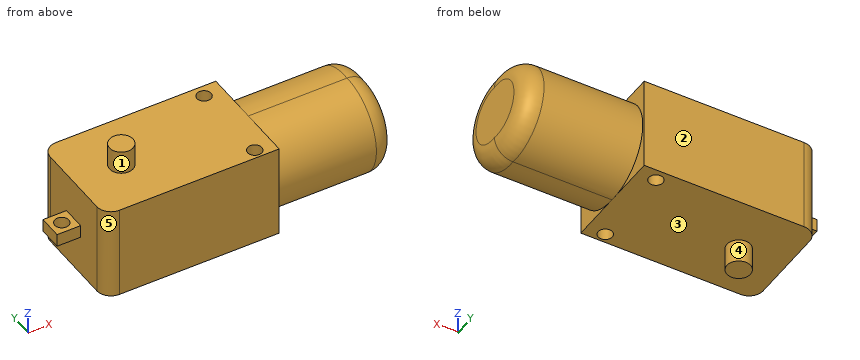
from build123d import *

# Parameters (mm, degrees)
SKETCH1_W           = 37
SKETCH1_H           = 22.5
BOSS_EXTRUDE1_DEPTH = 20
BOSS_EXTRUDE2_DEPTH = 25
SKETCH3_R           = 2.5
BOSS_EXTRUDE3_DEPTH = 5
BOSS_EXTRUDE4_START = 5
SKETCH4_R           = 2.5
BOSS_EXTRUDE4_DEPTH = 5
FILLET1_R           = 3
FILLET2_R           = 4
SKETCH5_W           = 2.75
SKETCH5_H           = 5
BOSS_EXTRUDE5_DEPTH = 5
SKETCH6_R           = 1.5
CUT_EXTRUDE1_DEPTH  = 2.75
SKETCH7_R           = 1.5
CUT_EXTRUDE2_DEPTH  = 78.76577433


with BuildPart() as part:
    # Sketch1 → Boss-Extrude1 (new body)
    with BuildSketch(Plane.XY):
        with Locations((-45.764100782, -13.75)):
            Rectangle(SKETCH1_W, SKETCH1_H)
    extrude(amount=-BOSS_EXTRUDE1_DEPTH)

    # Sketch2 → Boss-Extrude2 (add)
    with BuildSketch(Plane(origin=(-27.264100782, 0, 0), x_dir=(0, 0, -1), z_dir=(1, 0, 0))):
        with BuildLine():
            ThreePointArc((0.050125629, -14), (10, -24.462429423), (19.949874371, -14))
            ThreePointArc((19.949874371, -14), (10, -3), (0.050125629, -14))
        make_face()
    extrude(amount=BOSS_EXTRUDE2_DEPTH)

    # Sketch3 → Boss-Extrude3 (add)
    with BuildSketch(Plane.XY):
        with Locations((-54.264100782, -14)):
            Circle(SKETCH3_R)
    extrude(amount=BOSS_EXTRUDE3_DEPTH)

    # Sketch4 → Boss-Extrude4 (add)
    with BuildSketch(Plane(origin=(0, 0, -20), x_dir=(-1, 0, 0), z_dir=(0, 0, -1)).offset(BOSS_EXTRUDE4_START)):
        with Locations(Location((54.264100782, -14, 0), (0, 0, 180))):
            Circle(SKETCH4_R)
    extrude(amount=-BOSS_EXTRUDE4_DEPTH)

    # Fillet1
    fillet1_edges = [part.edges().sort_by_distance(p)[0] for p in [
        (-64.264100782, -2.5, -10),
        (-64.264100782, -25, -10),
    ]]
    fillet(fillet1_edges, radius=FILLET1_R)

    # Fillet2
    fillet2_edges = [part.edges().sort_by_distance(p)[0] for p in [
        (-2.264100782, -3, -10),
        (-2.264100782, -24.462429423, -10),
    ]]
    fillet(fillet2_edges, radius=FILLET2_R)

    # Sketch5 → Boss-Extrude5 (add)
    with BuildSketch(Plane.ZY.offset(64.264100782)):
        with Locations((-10, -13.75)):
            Rectangle(SKETCH5_W, SKETCH5_H)
    extrude(amount=BOSS_EXTRUDE5_DEPTH)

    # Sketch6 → Cut-Extrude1 (cut)
    with BuildSketch(Plane(origin=(0, 0, -11.375), x_dir=(-1, 0, 0), z_dir=(0, 0, -1))):
        with Locations((66.764100782, -13.75)):
            Circle(SKETCH6_R)
    extrude(amount=-CUT_EXTRUDE1_DEPTH, mode=Mode.SUBTRACT)

    # Sketch7 → Cut-Extrude2 (cut, through all)
    with BuildSketch(Plane(origin=(0, 0, -20), x_dir=(-1, 0, 0), z_dir=(0, 0, -1))):
        with Locations((31.264100782, -5)):
            Circle(SKETCH7_R)
        with Locations((31.264100782, -23)):
            Circle(SKETCH7_R)
    extrude(amount=-CUT_EXTRUDE2_DEPTH, mode=Mode.SUBTRACT)


solid = part.part
Verification items for the finished model (mm, model axes). Face numbers are marked on the shaded views. A direction names the side the tool comes from. Give positions to 0.01 mm unless a question says otherwise; leave off trailing zeros. Order: outer loops, then holes, each group sorted by start corner. A loop starts at its lowest first (then second) coordinate and runs counter-clockwise, first axis right, second up. Notation, with made-up numbers: M 71.25,13.25 L 77.25,13.25 A18 cw 77.25,34.25 Z; hole C 51,-24.75 d5. An arc over 180 degrees is marked long. Use one line per item in the form item = value. Start each with the question number.
Q1. Section check A-A (z = -10). Enter the section's corners in (x, y).
Q2. Mould release check, pull along X, two halves, no side actions. Record for the marked faces 3, 4 and 5: +X half, -X half, draft (parallel to the pull), parting line (faces both ways), or undercut.
Q3. Scan lines: line 1 along Z through (x, y) = (-38.5, -12); line 2 along X through (y, z) = (-13.25, -3.75); line 3 along Z through (x, y) = (-16.5, -14). Record each from-to range of solid material in increasing order. Write a range as [from, to].
Q4. Section check C-C (z = -15). Count the separate pieces of the cut face and the enclosed holes in it, then the cut area to 3 significant figures.
Q5. Access from +Z, -Z, +X, -X, +Y, -Y to the whole of each face (thin tool, end or side, straight path). Record for the marked faces 1 and 2.
Q6. Section check B-B (x = -60). Enter the section's corners in (y, z), then the cut area to 3 significant figures.
Q7. Section check D-D (z = 2.75). Enter the section's corners in (x, y).
Q8. Go/stop test with flat-tipped pins: pin 1 Ø3.5 at (x, y) = (-66.76, -13.75) entering from -Z (3 decimals); pin 2 Ø1 at (y, z) = (-6, -15) entering from -X; pin 3 Ø3 at (x, z) = (-67.5, -10) entering from -Y. Record where each tip stops, or that it passes through.
Evaluation:
q1.outline = M -69.26,-16.25 L -64.26,-16.25 L -64.26,-22 A3 ccw -61.26,-25 L -27.26,-25 L -27.26,-24.46 L -6.26,-24.46 A4 ccw -2.26,-20.46 L -2.26,-7 A4 ccw -6.26,-3 L -27.26,-3 L -27.26,-2.5 L -61.26,-2.5 A3 ccw -64.26,-5.5 L -64.26,-11.25 L -69.26,-11.25 Z; hole C -66.76,-13.75 d3; hole C -31.26,-23 d3; hole C -31.26,-5 d3
q2.face_3 = draft
q2.face_4 = parting line
q2.face_5 = -X half
q3.line_1 = [-20, 0]
q3.line_2 = [-64.26, -2.27]
q3.line_3 = [-19.95, -0.05]
q4.separate_pieces = 1
q4.enclosed_holes = 2
q4.area = 1,280 mm2
q5.face_1 = +Z
q5.face_2 = +Z, -Z, +X, -X, +Y
q6.outline = M -25,-20 L -2.5,-20 L -2.5,0 L -25,0 Z
q6.area = 450 mm2
q7.outline = C -54.26,-14 d5
q8.pin_1 = -11.375
q8.pin_2 = -64.26
q8.pin_3 = -16.25
